Geometry: see drawing. Coordinates: mm, zero at the bounding-box minimum. A direction names the side the tool comes from. Give positions to 0.01 mm unless a question says otherwise; leave off trailing zeros. Order: outer loops, then holes, each group sorted by start corner. A loop starts at its lowest first (then second) coordinate and runs counter-clockwise, first axis right, second up. Notation, with made-up numbers: (7, 41) - (54, 41) arc R30 cw to (54, 73) - close; hole circle Ø7 at (86, 67). An arc over 180 degrees is marked (long way). One line per item, written item: value. Start each with the question number.
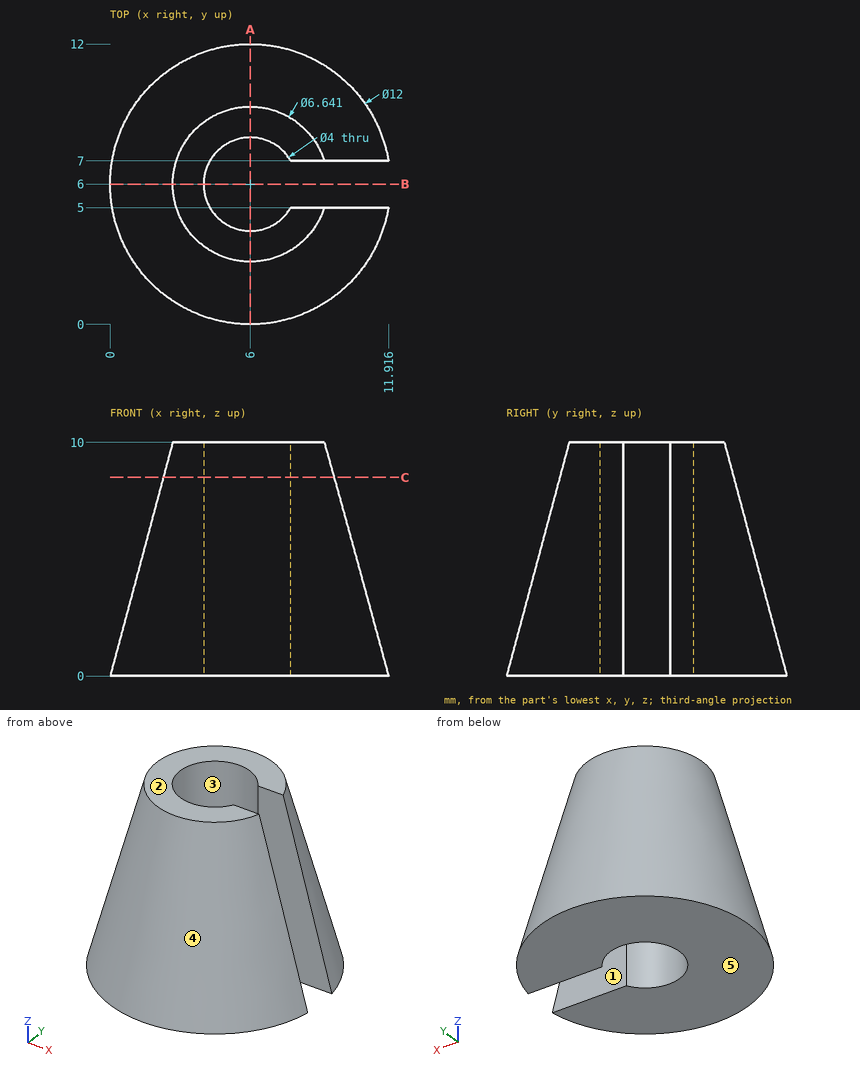
1. Contact query for flat-ended pins moving along their axis: pin 1 Ø3.5 at (x, z) = (9, 5.5) entering from +Y; pin 2 Ø3 at (x, y) = (3, 4) entering from +Z; pin 3 Ø5 at (x, z) = (4.5, 6.5) entering from +Y; pin 4 Ø6 at (y, z) = (10, 7) entering from +X. Output: stop coordinate, or through.
2. Ray query, L1, parallel to Y at x = 9, z = 7.75; L2, parallel to Y at x = 6.75, z = 2.75; L3, parallel to X at y = 6, z = 7. Return the intervals inside material, ascending.
3. Draft query along Y for the marked faces 3, 4 and 5. Return one class per face: pulls with the +Y half, pulls with the -Y half, needs draft (parallel to the pull), parting line crosses it, or undercut.
4. Section A-A on x = 6. Return the cut outline in (y, z).
5. Set-up query: the marked faces 1 and 2. Return all of +Z, -Z, +X, -X, +Y, -Y with unobstructed straight access to the full face (end or side cutting, diameter ignored); none if empty.
6. Section B-B on y = 6. Return the cut outline in (x, z), then the cut area to 3 significant figures.
7. Section C-C on z = 8.5. Return the cut outline in (x, y) (1 decimal).
Data:
1. pin 1: stops at y = 10.53
1. pin 2: stops at z = 10
1. pin 3: stops at y = 10.85
1. pin 4: stops at x = 10.32
2. L1: y = 3.47 to 5, 7 to 8.53
2. L2: y = 0.79 to 4.15, 7.85 to 11.21
2. L3: x = 1.88 to 4
3. face 3: undercut
3. face 4: parting line crosses it
3. face 5: needs draft
4. outline: (0, 0) - (4, 0) - (4, 10) - (2.68, 10) - close; (8, 0) - (12, 0) - (9.32, 10) - (8, 10) - close
5. face 1: +Z, -Z, +X
5. face 2: +Z, +X, -X, +Y, -Y
6. outline: (0, 0) - (4, 0) - (4, 10) - (2.68, 10) - close
6. area: 26.6 mm2
7. outline: (7.7, 5) arc R2 cw (long way) to (7.7, 7) - (9.6, 7) arc R3.7 ccw (long way) to (9.6, 5) - close
